```python
from build123d import *

# Parameters (mm, degrees)
SKETCH1_R                 = 38.1
SKETCH1_R_2               = 1.5875
BOSS_EXTRUDE1_DEPTH       = 10
BOSS_EXTRUDE2_DEPTH       = 80
RIB1_REACH                = 93.581
SKETCH3_WALL_W            = 227.849219062
SKETCH3_WALL_H            = 2
SKETCH5_R                 = 3.25
SKETCH5_R_2               = 4.25
CUT_EXTRUDE1_DEPTH        = 2
MIRROR2_COPY_1_REACH      = 93.581
MIRROR2_COPY_1_SKETCH_W   = 227.849219062
MIRROR2_COPY_1_SKETCH_H   = 2
MIRROR2_COPY_2_SKETCH_R   = 3.25
MIRROR2_COPY_2_SKETCH_R_2 = 4.25
MIRROR2_COPY_2_DEPTH      = 2
SKETCH12_R                = 1.625
CUT_EXTRUDE3_DEPTH        = 3
CUT_EXTRUDE4_DEPTH        = 3


with BuildPart() as part:
    # Sketch1 → Boss-Extrude1 (new body)
    with BuildSketch(Plane(origin=(0, 0, 0), x_dir=(1, 0, 0), z_dir=(0, 1, 0))):
        with Locations(Location((0, 0, 0), (0, 0, 270))):
            Circle(SKETCH1_R)
        with Locations(Location((0, 29.337, 0), (0, 0, 270))):
            Circle(SKETCH1_R_2, mode=Mode.SUBTRACT)
        with Locations(Location((25.406587271, -14.6685, 0), (0, 0, 270))):
            Circle(SKETCH1_R_2, mode=Mode.SUBTRACT)
        with Locations(Location((-25.406587271, -14.6685, 0), (0, 0, 270))):
            Circle(SKETCH1_R_2, mode=Mode.SUBTRACT)
    extrude(amount=BOSS_EXTRUDE1_DEPTH)


with BuildPart() as body_2:
    # Sketch2 → Boss-Extrude2 (new body)
    with BuildSketch(Plane(origin=(0, 10, 0), x_dir=(1, 0, 0), z_dir=(0, 1, 0))):
        with BuildLine():
            Line((-23.362837271, -11.128621162), (-13.453293635, 6.035211894))
            Line((-13.453293635, 6.035211894), (-12.703293635, 7.33425))
            Line((-12.703293635, 7.33425), (-11.953293635, 8.633288106))
            Line((-11.953293635, 8.633288106), (-2.04375, 25.797121162))
            ThreePointArc((-2.04375, 25.797121162), (-2.668939671, 26.241128995), (-3.200199346, 26.794092138))
            Line((-3.200199346, 26.794092138), (-24.804464136, -10.625592138))
            ThreePointArc((-24.804464136, -10.625592138), (-24.059954169, -10.809194941), (-23.362837271, -11.128621162))
        make_face()
        with BuildLine():
            Line((-12.15425553, 5.285211894), (-13.453293635, 6.035211894))
            Line((-13.453293635, 6.035211894), (-23.362837271, -11.128621162))
            ThreePointArc((-23.362837271, -11.128621162), (-22.7376476, -11.572628995), (-22.206387925, -12.125592138))
            Line((-22.206387925, -12.125592138), (-12.15425553, 5.285211894))
        make_face()
        with BuildLine():
            ThreePointArc((-21.319087271, -14.6685), (-21.547282212, -13.321866898), (-22.206387925, -12.125592138))
            Line((-22.206387925, -12.125592138), (-23.381660701, -14.161224299))
            ThreePointArc((-23.381660701, -14.161224299), (-23.334789686, -14.412939796), (-23.319087271, -14.6685))
            ThreePointArc((-23.319087271, -14.6685), (-26.663807692, -16.334949238), (-25.979736912, -12.661224299))
            Line((-25.979736912, -12.661224299), (-24.804464136, -10.625592138))
            ThreePointArc((-24.804464136, -10.625592138), (-28.502458276, -17.337439671), (-21.319087271, -14.6685))
        make_face()
        with BuildLine():
            Line((-24.362837271, -12.86067197), (-23.362837271, -11.128621162))
            ThreePointArc((-23.362837271, -11.128621162), (-24.059954169, -10.809194941), (-24.804464136, -10.625592138))
            Line((-24.804464136, -10.625592138), (-25.979736912, -12.661224299))
            ThreePointArc((-25.979736912, -12.661224299), (-25.151027067, -12.596702415), (-24.362837271, -12.86067197))
        make_face()
        with BuildLine():
            ThreePointArc((-22.206387925, -12.125592138), (-22.7376476, -11.572628995), (-23.362837271, -11.128621162))
            Line((-23.362837271, -11.128621162), (-24.362837271, -12.86067197))
            ThreePointArc((-24.362837271, -12.86067197), (-23.740138033, -13.411279579), (-23.381660701, -14.161224299))
            Line((-23.381660701, -14.161224299), (-22.206387925, -12.125592138))
        make_face()
        with BuildLine():
            ThreePointArc((4.0875, 29.337), (-1.346633102, 33.196305059), (-3.200199346, 26.794092138))
            Line((-3.200199346, 26.794092138), (-2.02492657, 28.829724299))
            ThreePointArc((-2.02492657, 28.829724299), (-0.255560204, 31.408797585), (2.0875, 29.337))
            ThreePointArc((2.0875, 29.337), (1.666449238, 28.079779579), (0.573149641, 27.329724299))
            Line((0.573149641, 27.329724299), (-0.602123135, 25.294092138))
            ThreePointArc((-0.602123135, 25.294092138), (2.668939671, 26.241128995), (4.0875, 29.337))
        make_face()
        with BuildLine():
            ThreePointArc((-3.200199346, 26.794092138), (-2.668939671, 26.241128995), (-2.04375, 25.797121162))
            Line((-2.04375, 25.797121162), (-1.04375, 27.52917197))
            ThreePointArc((-1.04375, 27.52917197), (-1.666449238, 28.079779579), (-2.02492657, 28.829724299))
            Line((-2.02492657, 28.829724299), (-3.200199346, 26.794092138))
        make_face()
        with BuildLine():
            Line((-1.04375, 27.52917197), (-2.04375, 25.797121162))
            ThreePointArc((-2.04375, 25.797121162), (-1.346633102, 25.477694941), (-0.602123135, 25.294092138))
            Line((-0.602123135, 25.294092138), (0.573149641, 27.329724299))
            ThreePointArc((0.573149641, 27.329724299), (-0.255560204, 27.265202415), (-1.04375, 27.52917197))
        make_face()
        with BuildLine():
            Line((-2.04375, 25.797121162), (-11.953293635, 8.633288106))
            Line((-11.953293635, 8.633288106), (-10.65425553, 7.883288106))
            Line((-10.65425553, 7.883288106), (-0.602123135, 25.294092138))
            ThreePointArc((-0.602123135, 25.294092138), (-1.346633102, 25.477694941), (-2.04375, 25.797121162))
        make_face()
        Polygon((-12.703293635, 7.33425), (-13.453293635, 6.035211894), (-12.15425553, 5.285211894), (-11.40425553, 6.58425), align=None)
        Polygon((-11.953293635, 8.633288106), (-12.703293635, 7.33425), (-11.40425553, 6.58425), (-10.65425553, 7.883288106), align=None)
        with BuildLine():
            Line((-10.65425553, 7.883288106), (-11.40425553, 6.58425))
            Line((-11.40425553, 6.58425), (21.866708433, -12.62475))
            ThreePointArc((21.866708433, -12.62475), (22.310716265, -11.999560329), (22.863679409, -11.468300654))
            Line((22.863679409, -11.468300654), (-10.65425553, 7.883288106))
        make_face()
        with BuildLine():
            Line((-11.40425553, 6.58425), (-12.15425553, 5.285211894))
            Line((-12.15425553, 5.285211894), (21.363679409, -14.066376865))
            ThreePointArc((21.363679409, -14.066376865), (21.547282212, -13.321866898), (21.866708433, -12.62475))
            Line((21.866708433, -12.62475), (-11.40425553, 6.58425))
        make_face()
        with BuildLine():
            ThreePointArc((22.863679409, -11.468300654), (22.310716265, -11.999560329), (21.866708433, -12.62475))
            Line((21.866708433, -12.62475), (23.59875924, -13.62475))
            ThreePointArc((23.59875924, -13.62475), (24.14936685, -13.002050762), (24.89931157, -12.64357343))
            Line((24.89931157, -12.64357343), (22.863679409, -11.468300654))
        make_face()
        with BuildLine():
            ThreePointArc((21.866708433, -12.62475), (21.547282212, -13.321866898), (21.363679409, -14.066376865))
            Line((21.363679409, -14.066376865), (23.39931157, -15.241649641))
            ThreePointArc((23.39931157, -15.241649641), (23.334789686, -14.412939796), (23.59875924, -13.62475))
            Line((23.59875924, -13.62475), (21.866708433, -12.62475))
        make_face()
        with BuildLine():
            Line((23.39931157, -15.241649641), (21.363679409, -14.066376865))
            ThreePointArc((21.363679409, -14.066376865), (25.104701229, -18.744836722), (29.494087271, -14.6685))
            ThreePointArc((29.494087271, -14.6685), (27.183314651, -10.987345824), (22.863679409, -11.468300654))
            Line((22.863679409, -11.468300654), (24.89931157, -12.64357343))
            ThreePointArc((24.89931157, -12.64357343), (26.690861039, -13.022809526), (27.494087271, -14.6685))
            ThreePointArc((27.494087271, -14.6685), (25.695955743, -16.735846642), (23.39931157, -15.241649641))
        make_face()
    extrude(amount=BOSS_EXTRUDE2_DEPTH)

    # Sketch3 wall → Rib1 (add, up to next)
    with BuildSketch(Plane(origin=(0.022296069, 90, 14.367438433), x_dir=(-0.999900512002, 0, 0.014105534336), z_dir=(0.014105534336, 0, 0.999900512002)), mode=Mode.PRIVATE) as rib1_sk1:
        with Locations((0, 1)):
            Rectangle(SKETCH3_WALL_W, SKETCH3_WALL_H)
    rib1_tool1 = extrude(rib1_sk1.sketch, amount=-RIB1_REACH, mode=Mode.PRIVATE) - body_2.part
    rib1 = rib1_tool1.solids().sort_by_distance((0.022296069, 90, 14.367438433))[0]
    add(rib1)

    # Sketch5 → Cut-Extrude1 (cut)
    with BuildSketch(Plane.XZ.offset(-88)):
        with Locations(Location((0.684201738, 8.477927826, 0), (0, 0, 270))):
            Circle(SKETCH5_R)
        with Locations(Location((-8.976052299, 5.209978634, 0), (0, 0, 270))):
            Circle(SKETCH5_R_2)
    cut_extrude1 = extrude(amount=-CUT_EXTRUDE1_DEPTH, mode=Mode.SUBTRACT)

    # Mirror1: Rib1, Cut-Extrude1 across plane
    add(rib1.mirror(Plane.ZX.offset(50)))
    add(cut_extrude1.mirror(Plane.ZX.offset(50)), mode=Mode.SUBTRACT)

    # Mirror2: Rib1, Cut-Extrude1 across plane
    add(rib1.mirror(Plane(origin=(0, 0, 0), x_dir=(0.8660254037844597, 0, 0.49999999999996353), z_dir=(0.49999999999996314, 0, -0.8660254037844598))))
    add(cut_extrude1.mirror(Plane(origin=(0, 0, 0), x_dir=(0.8660254037844597, 0, 0.49999999999996353), z_dir=(0.49999999999996314, 0, -0.8660254037844598))), mode=Mode.SUBTRACT)

    # Mirror2 copy 1 sketch → Mirror2 copy 1 (add, up to next)
    with BuildSketch(Plane(origin=(12.453714705, 10, -7.164410254), x_dir=(-0.48773450493214454, 0, -0.8729920118187576), z_dir=(0.8729920118187576, 0, -0.48773450493214465)), mode=Mode.PRIVATE) as mirror2_copy_1_sk1:
        with Locations((0, 1)):
            Rectangle(MIRROR2_COPY_1_SKETCH_W, MIRROR2_COPY_1_SKETCH_H)
    mirror2_copy_1_tool1 = extrude(mirror2_copy_1_sk1.sketch, amount=-MIRROR2_COPY_1_REACH, mode=Mode.PRIVATE) - body_2.part
    add(mirror2_copy_1_tool1.solids().sort_by_distance((12.453714705, 10, -7.164410254))[0])

    # Mirror2 copy 2 sketch → Mirror2 copy 2 (cut)
    with BuildSketch(Plane(origin=(0, 12, 0), x_dir=(0.5000000000000736, 0, 0.8660254037843962), z_dir=(0, 1, 0))):
        with Locations(Location((0.684201738, 8.477927826, 0), (0, 0, 270))):
            Circle(MIRROR2_COPY_2_SKETCH_R)
        with Locations(Location((-8.976052299, 5.209978634, 0), (0, 0, 270))):
            Circle(MIRROR2_COPY_2_SKETCH_R_2)
    extrude(amount=-MIRROR2_COPY_2_DEPTH, mode=Mode.SUBTRACT)

    # Sketch12 → Cut-Extrude3 (cut)
    with BuildSketch(Plane(origin=(-0.75, 0, 1.299038106), x_dir=(0.8660254037844608, 0, 0.49999999999996164), z_dir=(-0.49999999999996175, 0, 0.8660254037844609))):
        with Locations((-2.197056325, 80.875)):
            Circle(SKETCH12_R)
        with Locations((-2.197056325, 19.125)):
            Circle(SKETCH12_R)
        with Locations((20.802943675, 19.125)):
            Circle(SKETCH12_R)
        with Locations((20.802943675, 80.875)):
            Circle(SKETCH12_R)
    extrude(amount=-CUT_EXTRUDE3_DEPTH, mode=Mode.SUBTRACT)

    # Sketch13 → Cut-Extrude4 (cut)
    with BuildSketch(Plane(origin=(0.75, 0, -1.299038106), x_dir=(-0.8660254037844608, 0, -0.49999999999996164), z_dir=(0.49999999999996175, 0, -0.8660254037844609))):
        Polygon((6.197056325, 76.875), (6.197056325, 23.125), (-1.802943675, 23.125), (-1.802943675, 15.125), (-16.802943675, 15.125), (-16.802943675, 23.125), (-24.802943675, 23.125), (-24.802943675, 76.875), (-16.802943675, 76.875), (-16.802943675, 84.875), (-1.802943675, 84.875), (-1.802943675, 76.875), align=None)
    extrude(amount=-CUT_EXTRUDE4_DEPTH, mode=Mode.SUBTRACT)


solid = body_2.part
```
Check sheet for the modelled part. Datum: model origin and axes. Units: mm. A direction names the side the tool comes from. Give positions to 0.01 mm unless a question says otherwise; leave off trailing zeros. Order: outer loops, then holes, each group sorted by start corner. A loop starts at its lowest first (then second) coordinate and runs counter-clockwise, first axis right, second up. Notation, with made-up numbers: (10.5, 25) -> (50.5, 25) arc R9 ccw to (50.5, 31) -> close; hole circle Ø5 at (-12, 7). An arc over 180 degrees is marked (long way). Use CSV: the item, a comma, the result in double quotes. Start each with the question number.
1) Set-up check for faces 1 (the face through (1.572, 19.181, 0.883)), 2 (the face through (1.66, 11.014, 5.378)): record each of +Z, -Z, +X, -X, +Y, -Y from which the full face is reachable in a straight line by a thin tool's end or side.
2) Sectioned sample at B-B, the plane x = 7. Record the boundary of the cut face in (y, z) (1 decimal).
3) Go/stop test with flat-tipped pins: P1, Ø3, axis at y = 26, z = -4.5, coming from the -X side; P2, Ø7, axis at x = -8.98, z = 5.21, coming from the -Y side; P3, Ø10, axis at x = -19, y = 48, coming from the -Z side; P4, Ø5, axis at y = 60.5, z = -1.5, coming from the +X side. Record where each tip stops, or that it passes through.
4) Mould release check, pull along Z, two halves, no side actions. Record for faces 3 (the face through (-1.253, 88.986, -14.432)), 4 (the face through (1.572, 80.931, 0.883)), 5 (the face through (14.562, 80.819, 8.383)), 6 (the face through (-3, 10, 1)): released by +Z, released by -Z, zero draft, split by the parting line, or undercut.
5) Sectioned sample at C-C, the plane z = 3.5. Record the boundary of the cut face in (x, y) (1 decimal).
6) Sectioned sample at D-D, the plane z = -18. Record the boundary of the cut face in (x, y).
7) Sectioned sample at A-A, the plane y = 70. Record the boundary of the cut face in (x, z) (1 decimal), plus the area to 3 significant figures.
8) Material ranges on line 1 (Z direction, x = 0, y = 58); line 2 (Y direction, x = 8.5, z = 3); line 3 (X direction, y = 36, z = 14), recorded low to high. Write a range as from..to.
Recorded:
1,face 1,"+Z, +X"
1,face 2,"+Y, -Y"
2,outline,"(10, -16.9) -> (12, -16.9) -> (12, -6.8) -> (10, -6.8) -> close; (10, -0.5) -> (12, -0.5) -> (12, 2.3) -> (15.1, 2.3) -> (15.1, 5.8) -> (12, 5.8) -> (12, 14.3) -> (10, 14.3) -> close; (84.9, 2.3) -> (88, 2.3) -> (88, -0.5) -> (90, -0.5) -> (90, 14.3) -> (88, 14.3) -> (88, 5.8) -> (84.9, 5.8) -> close; (88, -16.9) -> (90, -16.9) -> (90, -6.8) -> (88, -6.8) -> close"
3,P1,"x = -16.94"
3,P2,"through"
3,P3,"z = -8.09"
3,P4,"x = -4.85"
4,face 3,"undercut"
4,face 4,"released by +Z"
4,face 5,"released by -Z"
4,face 6,"zero draft"
5,outline,"(-20.7, 10) -> (-12.9, 10) -> (-12.9, 12) -> (-17.2, 12) -> (-17.2, 88) -> (-12.9, 88) -> (-12.9, 90) -> (-20.7, 90) -> close; (-5.1, 10) -> (18.4, 10) -> (18.4, 12) -> (9.1, 12) -> (9.1, 15.1) -> (3.1, 15.1) -> (3.1, 12) -> (-5.1, 12) -> close; (-5.1, 88) -> (3.1, 88) -> (3.1, 84.9) -> (9.1, 84.9) -> (9.1, 88) -> (18.4, 88) -> (18.4, 90) -> (-5.1, 90) -> close"
6,outline,"(-8.28, 10) -> (6.4, 10) -> (6.4, 12) -> (-4.81, 12) -> (-4.81, 88) -> (6.4, 88) -> (6.4, 90) -> (-8.28, 90) -> close"
7,outline,"(-24.8, 10.6) -> (-3.2, -26.8) arc R4.1 ccw (long way) to (-0.6, -25.3) -> (-10.7, -7.9) -> (-4.6, -4.4) -> (-6.1, -1.8) -> (-12.2, -5.3) -> (-22.2, 12.1) arc R4.1 ccw (long way) to start; (20.7, 13.7) -> (22.2, 11.1) -> (22.9, 11.5) arc R4.1 ccw (long way) to (21.4, 14.1) -> close; hole circle Ø4.2 at (-25.4, 14.7); hole circle Ø4.2 at (0, -29.3); hole circle Ø4.2 at (25.4, 14.7)"
7,area,"267 mm2"
8,line 1,"-33.42..-31.42, -27.25..-25.25"
8,line 2,"10..12, 88..90"
8,line 3,"-29.44..-27.38, -23.43..-21.37, 21.25..23.43, 27.38..29.44"
